Autodesk Inventor part; units mm, degrees
ref_plane "YZ Plane" through (0, 0, 0) normal (1, 0, 0) x (0, 1, 0)
ref_plane "XZ Plane" through (0, 0, 0) normal (0, 1, 0) x (-1, 0, 0)
ref_plane "XY Plane" through (0, 0, 0) normal (0, 0, 1) x (1, 0, 0)
sketch "Sketch1" plane through (0, 0, 0) normal (0, 0, 1) x (1, 0, 0)
  line L0 (-47.9201, 83) -> (47.9201, 83)
  line L1 (47.9201, 83) -> (95.8401, 0)
  line L2 (95.8401, 0) -> (47.9201, -83)
  line L3 (47.9201, -83) -> (-47.9201, -83)
  line L4 (-47.9201, -83) -> (-95.8401, 0)
  line L5 (-95.8401, 0) -> (-47.9201, 83)
  point P0 (0, 0)
  point P1 (0, 0)
  dimension "d0" = 166
extrude "Extrusion1" add sketch "Sketch1" along normal blind 2
sketch "Sketch3" plane through (0, 0, 2) normal (0, 0, 1) x (1, 0, 0)
  line L0 (47.9201, 83) -> (-47.9201, 83)
  line L1 (-47.9201, 83) -> (-95.8401, 0)
  line L2 (-95.8401, 0) -> (-47.9201, -83)
  line L3 (-47.9201, -83) -> (47.9201, -83)
  line L4 (47.9201, -83) -> (95.8401, 0)
  line L5 (95.8401, 0) -> (47.9201, 83)
  line L6 (-95.8401, 83) -> (95.8401, 83)
  line L7 (95.8401, 83) -> (95.8401, -83)
  line L8 (95.8401, -83) -> (-95.8401, -83)
  line L9 (-95.8401, -83) -> (-95.8401, 83)
  line L10 (-95.8401, 83) -> (95.8401, -83) construction
  line L11 (95.8401, 83) -> (-95.8401, -83) construction
  point P0 (0, 0)
  dimension "d3" = 191.6803
  dimension "d4" = 166
properties part number "Frosted Top v1"
Can you work these out from the model? Positions are in its coordinate system, mm. Round coordinates to 2 decimals unless told otherwise and drop trailing zeros. Loops run counter-clockwise (first coordinate to the right, second up) from the corner with the lowest first, then second, coordinate; pieces in that order, holes last. Notation, with made-up numbers: M 77.25,-13.75 L 133.25,-13.75 A11 ccw 133.25,4.25 Z; hole C 8.5,31.5 d2. An arc over 180 degrees is marked long. Answer in a Markdown table with one row per item.
1. If we section it at B-B, the plane x = -54.5: Please give me the cut outline in (y, z).
Established:
| item | result |
|---|---|
| outline | M -71.6,0 L 71.6,0 L 71.6,2 L -71.6,2 Z |
2. If we section it at C-C, the plane y = 68: Please give me the cut outline in (x, z), plus the area to 3 significant figures.
Established:
| item | result |
|---|---|
| outline | M -56.58,0 L 56.58,0 L 56.58,2 L -56.58,2 Z |
| area | 226 mm² |
3. I'm going to push a flat-ended pin straight in: pin 1 Ø1 at (y, z) = (18, 0.5) entering from -X. Where does the tip first touch, or does it pass through?
Established:
| item | result |
|---|---|
| pin 1 | x = -85.74 |
4. Please list where these lines run through material, in increasing order: line 1 (X direction, y = 28, z = 0.65); line 2 (X direction, y = -38.5, z = 0.95); line 3 (Y direction, x = 87, z = 0.6). Write a range as from..to.
Established:
| item | result |
|---|---|
| line 1 | -79.67..79.67 |
| line 2 | -73.61..73.61 |
| line 3 | -15.31..15.31 |
5. If we section it at A-A, the plane z = 1.2: Please give me the cut outline in (x, y), plus the area to 3 significant figures.
Established:
| item | result |
|---|---|
| outline | M -95.84,0 L -47.92,-83 L 47.92,-83 L 95.84,0 L 47.92,83 L -47.92,83 Z |
| area | 23,900 mm² |
